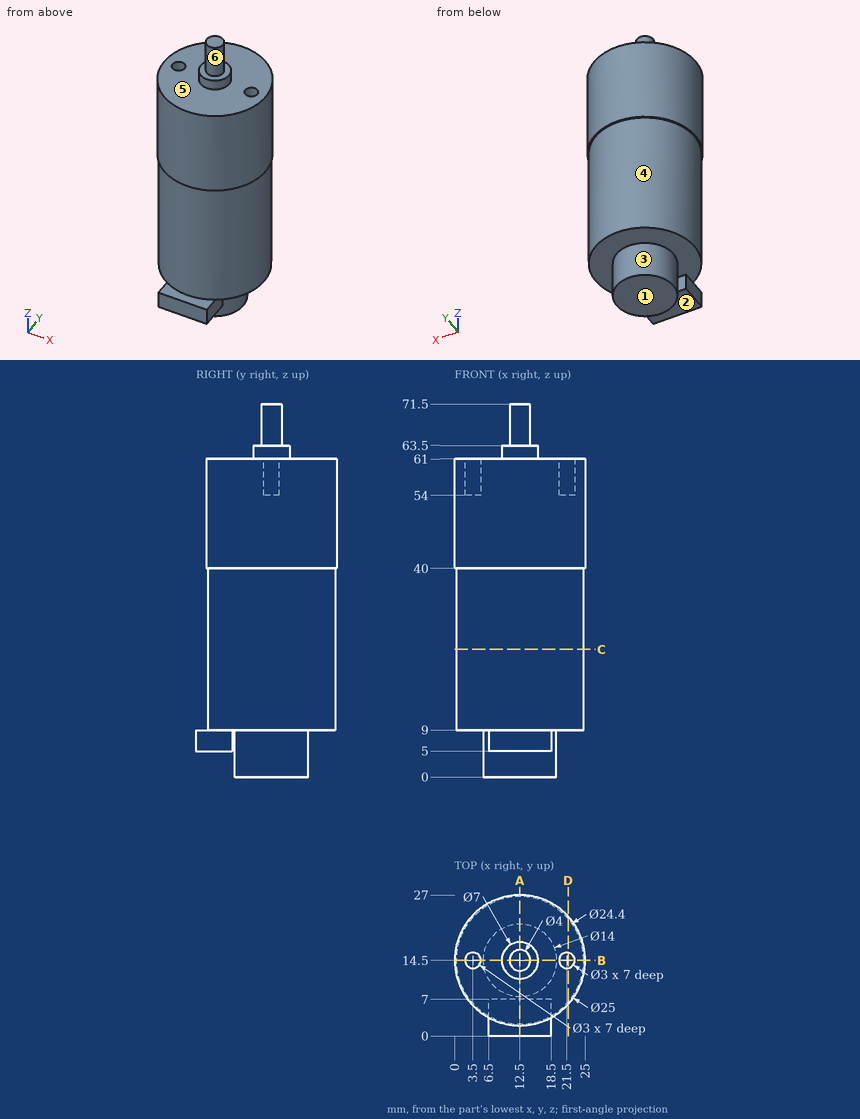
Answer from the drawing. Dimensions are ordinates in mm from the lowest x, y and z of the part. A direction names the side the tool comes from. Give positions to 0.01 mm unless a question says otherwise; leave off trailing zeros. Loops run counter-clockwise (first coordinate to the right, second up) from the corner with the lowest first, then second, coordinate; pieces in that order, holes last. Notation, with made-up numbers: M 46.25,-7 L 80.25,-7 A21 ccw 80.25,16 Z; hole C -19,70.5 d4. An arc over 180 degrees is marked long. One line per item, written item: value.
Q1. A cutting plane is placed at B-B on y = 14.5. Determine the outline of the cut face in (x, z).
Working result:
outline: M 0,40 L 0.3,40 L 0.3,9 L 5.5,9 L 5.5,0 L 19.5,0 L 19.5,9 L 24.7,9 L 24.7,40 L 25,40 L 25,61 L 23,61 L 23,54 L 20,54 L 20,61 L 16,61 L 16,63.5 L 14.5,63.5 L 14.5,71.5 L 10.5,71.5 L 10.5,63.5 L 9,63.5 L 9,61 L 5,61 L 5,54 L 2,54 L 2,61 L 0,61 Z
Q2. Determine the mould class of the marked faces 4, 5 and 6 for opening direction Z: +Z half, -Z half, draft (parallel to the pull), parting line (faces both ways), or undercut.
Working result:
face 4: undercut
face 5: +Z half
face 6: draft
Q3. Find the intervals of material crossed by line 1 (Z direction, x = 17, y = 3); line 2 (Z direction, x = 13.5, y = 8.25); line 3 (Y direction, x = 3.5, z = 55.5), in increasing order. Write a range as from..to.
Working result:
line 1: z = 5..9, 40..61
line 2: z = 0..61
line 3: y = 5.83..13, 16..23.17
Q4. A cutting plane is placed at D-D on x = 21.75. Determine the outline of the cut face in (y, z).
Working result:
outline: M 6.09,40 L 6.55,40 L 6.55,9 L 22.45,9 L 22.45,40 L 22.91,40 L 22.91,61 L 15.98,61 L 15.98,54 L 13.02,54 L 13.02,61 L 6.09,61 Z
Q5. Flat-ended cylindrical pins translate along their axes: P1, Ø2, axis at x = 13, y = 3, coming from the -Z side; P2, Ø2.5, axis at x = 21.5, y = 14.5, coming from the -Z side; P3, Ø12, axis at x = 20, z = 40.5, coming from the -Y side. Find the tip coordinate at first contact, or state that the pin passes through.
Working result:
P1: stops at z = 5
P2: stops at z = 9
P3: stops at y = 2.09
Q6. A cutting plane is placed at A-A on x = 12.5. Determine the outline of the cut face in (y, z), then the cut area to 3 significant figures.
Working result:
outline: M 0,5 L 7,5 L 7,9 L 7.5,9 L 7.5,0 L 21.5,0 L 21.5,9 L 26.7,9 L 26.7,40 L 27,40 L 27,61 L 18,61 L 18,63.5 L 16.5,63.5 L 16.5,71.5 L 12.5,71.5 L 12.5,63.5 L 11,63.5 L 11,61 L 2,61 L 2,40 L 2.3,40 L 2.3,9 L 0,9 Z
area: 1,480 mm^2
Q7. For the marked faces 1, 2 and 3, determine the directions among +Z, -Z, +X, -X, +Y, -Y from which every point of the face is accessible in a straight line to the end or side of a thin tool.
Working result:
face 1: -Z, +X, -X, +Y, -Y
face 2: -Z, +X, -X, -Y
face 3: -Z
Q8. A cutting plane is placed at C-C on z = 24.5. Determine the outline of the cut face in (x, y), then the cut area to 3 significant figures.
Working result:
outline: C 12.5,14.5 d24.4
area: 468 mm^2
